Work out the finished part from the listing and answer in its coordinate system (mm). Round coordinates to 2 decimals unless told otherwise and drop trailing zeros. Order: outer loops, then holes, each group sorted by start corner. A loop starts at its lowest first (then second) coordinate and runs counter-clockwise, first axis right, second up. Notation, with made-up numbers: (-23.5, 42) - (27.5, 42) arc R21 ccw to (27.5, 66) - close; hole circle Ø7 at (-10.75, 50.25). An arc over 180 degrees is marked (long way). Put each result on its own line as item: value.
Autodesk Inventor part; units mm, degrees
ref_plane "YZ Plane" through (0, 0, 0) normal (1, 0, 0) x (0, 1, 0)
ref_plane "XZ Plane" through (0, 0, 0) normal (0, 1, 0) x (-1, 0, 0)
ref_plane "XY Plane" through (0, 0, 0) normal (0, 0, 1) x (1, 0, 0)
sketch "Sketch1" plane through (0, 0, 0) normal (0, 1, 0) x (-1, 0, 0)
  line L0 (0, 0) -> (31.75, 0)
  line L1 (31.75, 0) -> (31.75, -25.4)
  line L2 (31.75, -25.4) -> (0, -25.4)
  line L3 (0, -25.4) -> (0, 0)
  circle A0 centre (26.67, -5.08) radius 1.27
  circle A1 centre (26.67, -20.32) radius 1.27
  circle A2 centre (5.08, -20.32) radius 1.27
  circle A3 centre (5.08, -5.08) radius 1.27
  dimension "d0" = 31.75
  dimension "d1" = 25.4
  dimension "d2" = 2.54
  dimension "d3" = 2.54
  dimension "d4" = 2.54
  dimension "d5" = 2.54
  dimension "d6" = 15.24
  dimension "d7" = 21.59
  dimension "d8" = 0
  dimension "d9" = 0
  dimension "d10" = 0
  dimension "d11" = 0
  dimension "d12" = 5.08
  dimension "d13" = 5.08
extrude "Extrusion1" add sketch "Sketch1" along normal blind 3.175
sketch "Sketch2" plane through (0, 3.175, 0) normal (0, 1, 0) x (1, 0, 0)
  circle A0 centre (-15.875, 16.51) radius 2.159
  line L0 (0, 25.4) -> (-31.75, 25.4)
  circle A1 centre (-15.875, 8.4836) radius 2.159
  line L1 (0, 0) -> (0, 25.4)
  dimension "d16" = 4.318
  dimension "d17" = 8.89
  dimension "d18" = 4.318
  dimension "d19" = 8.0264
  dimension "d20" = 15.875
  dimension "d21" = 15.875
extrude "Extrusion2" cut sketch "Sketch2" against normal through all
properties part number "IMU Mount"
1) A cutting plane is placed at B-B on z = -16.51. Write down the section's boundary in (x, y) (3 decimals), then the cut area to 3 significant figures.
Findings below:
outline: (-31.75, 0) - (-18.034, 0) - (-18.034, 3.175) - (-31.75, 3.175) - close; (-13.716, 0) - (0, 0) - (0, 3.175) - (-13.716, 3.175) - close
area: 87.1 mm2
2) A cutting plane is placed at D-D on y = 2.3. Write down the section's boundary in (x, z) (3 decimals).
Findings below:
outline: (-31.75, -25.4) - (0, -25.4) - (0, 0) - (-31.75, 0) - close; hole circle Ø2.54 at (-26.67, -20.32); hole circle Ø2.54 at (-26.67, -5.08); hole circle Ø4.318 at (-15.875, -16.51); hole circle Ø4.318 at (-15.875, -8.484); hole circle Ø2.54 at (-5.08, -20.32); hole circle Ø2.54 at (-5.08, -5.08)
3) For a pull along Z with two mould halves and no side action, classify faces 1 (the cylindrical face through (-25.734, 1.565, -21.178)), 2 (the flat face through (-31.75, 2, -13)), 3 (the flat face through (-16, 2, -25.4)), 4 (the flat face through (-16, 2, 0)) as pulls with the +Z half, pulls with the -Z half, needs draft (parallel to the pull), parting line crosses it, or undercut.
Findings below:
face 1: undercut
face 2: needs draft
face 3: pulls with the -Z half
face 4: pulls with the +Z half
4) Straight lines are drawn through the part: L1, parallel to Z at x = -5.08, y = 1.35; L2, parallel to X at y = 0.75, z = -19.5; L3, parallel to Z at x = -27, y = 1.7. For each, find the intervals that lie inside material, in ascending order. Write a range as from..to.
Findings below:
L1: z = -25.4..-21.59, -19.05..-6.35, -3.81..0
L2: x = -31.75..-27.64, -25.7..-6.05, -4.11..0
L3: z = -25.4..-21.55, -19.09..-6.31, -3.85..0
5) A cutting plane is placed at A-A on z = -5.08. Write down the section's boundary in (x, y) (3 decimals).
Findings below:
outline: (-31.75, 0) - (-27.94, 0) - (-27.94, 3.175) - (-31.75, 3.175) - close; (-25.4, 0) - (-6.35, 0) - (-6.35, 3.175) - (-25.4, 3.175) - close; (-3.81, 0) - (0, 0) - (0, 3.175) - (-3.81, 3.175) - close
6) Given pin 1 Ø1 at (x, z) = (-20, -14) entering from -Y, flat-ended and moving along its own axis, determine where the tip first touches the part or whether it passes through.
Findings below:
pin 1: stops at y = 0
7) A cutting plane is placed at C-C on x = -26.67. Write down the section's boundary in (y, z) (3 decimals), then the cut area to 3 significant figures.
Findings below:
outline: (0, -25.4) - (3.175, -25.4) - (3.175, -21.59) - (0, -21.59) - close; (0, -19.05) - (3.175, -19.05) - (3.175, -6.35) - (0, -6.35) - close; (0, -3.81) - (3.175, -3.81) - (3.175, 0) - (0, 0) - close
area: 64.5 mm2
